Autodesk Inventor part; units mm, degrees
ref_plane "YZ Plane" through (0, 0, 0) normal (1, 0, 0) x (0, 1, 0)
ref_plane "XZ Plane" through (0, 0, 0) normal (0, 1, 0) x (-1, 0, 0)
ref_plane "XY Plane" through (0, 0, 0) normal (0, 0, 1) x (1, 0, 0)
sketch "スケッチ1" plane through (0, 0, 0) normal (0, 0, 1) x (1, 0, 0)
  line L0 (-9, -27.5) -> (9, -27.5)
  line L1 (9, -27.5) -> (9, 27.5)
  line L2 (9, 27.5) -> (-9, 27.5)
  line L3 (-9, 27.5) -> (-9, -27.5)
  line L4 (-9, -27.5) -> (9, 27.5) construction
  line L5 (9, -27.5) -> (-9, 27.5) construction
  point P0 (0, 0)
  dimension "d0" = 18
  dimension "d1" = 55
extrude "プレート1" add sketch "スケッチ1" along normal blind 1.6
sketch "スケッチ2" plane through (9, -25.9, 0) normal (0, -1, 0) x (1, 0, 0)
  line L0 (-18, 0) -> (0, 0)
  line L1 (0, 0) -> (0, 11)
  line L2 (0, 11) -> (-18, 11)
  line L3 (-18, 11) -> (-18, 0)
edge flange "フランジ1" height 11 angle 90 thickness 1.6 bend radius 1.6 thickness toward (0, -1, 0) relief tear relief width 1.6 relief depth 0.8 edges at (0, -27.5, 1.6) wall of the first edge with corners at (-9, -25.9, 0) (9, -25.9, 0) (9, -25.9, 11) (-9, -25.9, 11)
bend "曲げ1"
corner "コーナー1"
sketch "スケッチ3" plane through (0, 0, 1.6) normal (0, 0, 1) x (1, 0, 0)
  line L0 (-9, 27.5) -> (9, 27.5)
  point P0 (0, 0)
  point P1 (0, 22.5)
  point P2 (0, -7.5)
  dimension "d13" = 5
  dimension "d14" = 30
hole "穴1" at (0, 22.5, 1.6) at (0, -7.5, 1.6) direction (0, 0, -1) diameter 4.3 end through all
sketch "スケッチ4" plane through (-9, -27.5, 11) normal (0, -1, 0) x (1, 0, 0)
  line L0 (0, 0) -> (18, 0)
  line L1 (18, 0) -> (18, -7.8)
  line L2 (0, -7.8) -> (0, 0)
  point P0 (9, -11)
  point P1 (14, -4)
  point P2 (4, -4)
  dimension "d22" = 4
  dimension "d40" = 4
  dimension "d41" = 4
hole "穴2" at (5, -27.5, 7) at (-5, -27.5, 7) direction (0, 1, 0) diameter 2.459 end through all
fillet "コーナーR1" radius 2 3 edges at (9, -26.7, 11) (-9, 27.5, 0.8) (9, 27.5, 0.8)
fillet "コーナーR2" radius 2 1 edges at (-9, -26.7, 11)
equation "\"d20\" = Thickness"
equation "\"d30\" = Thickness"
equation "\"d2\" = Thickness"
equation "\"d3\" = BendReliefWidth"
equation "\"d4\" = BendReliefDepth"
equation "\"d5\" = MinimumRemnant"
equation "\"d6\" = TransitionRadius"
equation "\"d9\" = BendRadius"
equation "\"d10\" = CornerReliefSize"
equation "\"d11\" = GapSize"
equation "\"d12\" = JacobiRadiusSize"
equation "\"BendRadius\" = Thickness"
equation "\"BendReliefWidth\" = Thickness"
equation "\"BendReliefDepth\" = 0.5 * Thickness"
equation "\"CornerReliefSize\" = 4 * Thickness"
equation "\"MinimumRemnant\" = 2 * Thickness"
equation "\"TransitionRadius\" = BendRadius"
equation "\"JacobiRadiusSize\" = BendRadius"
equation "\"GapSize\" = Thickness"
properties part number "steel_plate7" material "鋼、炭素鋼"
CAD build for the part. Positions are in the model's coordinates, mm. A direction names the side the tool comes from. Coordinates: 2 decimals unless noted, no trailing zeros. Order: outer loops, then holes, each group sorted by start corner. A loop starts at its lowest first (then second) coordinate and runs counter-clockwise, first axis right, second up.
Item 1: 3-axis set-ups, long thin cutter, end or side, ignore diameter. For faces 4 (the face through (0, 2, 0)), 5 (the face through (0, -25.9, 7)): which of +Z, -Z, +X, -X, +Y, -Y reach the whole face in a straight line?
Check sheet entries:
face 4: -Z, +X, -X, +Y, -Y
face 5: +Z, +X, -X, +Y
Item 2: Two-plate mould, pull along Z, no slides. Class faces 1 (the face through (9, -5, 1)), 2 (the face through (-8.4, -26.71, 10.43)), 3 (the face through (-3.91, -26.69, 6.43)): +Z half, -Z half, draft (parallel to the pull), parting line (faces both ways), or undercut.
Check sheet entries:
face 1: draft
face 2: +Z half
face 3: undercut
Item 3: Band-saw the part on D-D on x = 3. List the corners of the cut face in (y, z), plus the area to 3 significant figures.
Check sheet entries:
outline: (-27.5, 3.2) arc R3.2 ccw to (-24.3, 0) - (27.5, 0) - (27.5, 1.6) - (-24.3, 1.6) arc R1.6 cw to (-25.9, 3.2) - (-25.9, 11) - (-27.5, 11) - close
area: 101 mm2
Item 4: Band-saw the part on C-C on x = 0. List the corners of the cut face in (y, z).
Check sheet entries:
outline: (-27.5, 3.2) arc R3.2 ccw to (-24.3, 0) - (-9.65, 0) - (-9.65, 1.6) - (-24.3, 1.6) arc R1.6 cw to (-25.9, 3.2) - (-25.9, 11) - (-27.5, 11) - close; (-5.35, 0) - (20.35, 0) - (20.35, 1.6) - (-5.35, 1.6) - close; (24.65, 0) - (27.5, 0) - (27.5, 1.6) - (24.65, 1.6) - close
Item 5: Band-saw the part on A-A on x = -5. List the corners of the cut face in (y, z).
Check sheet entries:
outline: (-27.5, 3.2) arc R3.2 ccw to (-24.3, 0) - (27.5, 0) - (27.5, 1.6) - (-24.3, 1.6) arc R1.6 cw to (-25.9, 3.2) - (-25.9, 5.77) - (-27.5, 5.77) - close; (-27.5, 8.23) - (-25.9, 8.23) - (-25.9, 11) - (-27.5, 11) - close
Item 6: Pin check, flat tips, straight feed: pin 1 Ø7 at (x, y) = (0, 22.5) entering from +Z; pin 2 Ø2 at (x, z) = (5, 7) entering from +Y; pin 3 Ø3 at (x, z) = (-6, 1.5) entering from -Y; pin 4 Ø4 at (x, z) = (-4, 8) entering from +Y. Stop position of each tip, or through.
Check sheet entries:
pin 1: stops at z = 1.6
pin 2: passes through
pin 3: stops at y = -27.49
pin 4: stops at y = -25.9
Item 7: Drill centre lines: L1, parallel to X at y = -26.8, z = 7; L2, parallel to Z at x = 7.25, y = 10; L3, parallel to Y at x = 8, z = 10.25. Where is each one in solid material? Low to high.
Check sheet entries:
L1: x = -9 to -6.23, -3.77 to 3.77, 6.23 to 9
L2: z = 0 to 1.6
L3: y = -27.5 to -25.9
Item 8: Band-saw the part on B-B on y = -7.5. List the corners of the cut face in (x, z), plus the area to 3 significant figures.
Check sheet entries:
outline: (-9, 0) - (-2.15, 0) - (-2.15, 1.6) - (-9, 1.6) - close; (2.15, 0) - (9, 0) - (9, 1.6) - (2.15, 1.6) - close
area: 21.9 mm2
